Answer from the drawing. Dimensions are ordinates in mm from the lowest x, y and z of the part. Coordinates: 2 decimals unless noted, no trailing zeros. Order: outer loops, then holes, each group sorted by start corner. A loop starts at its lowest first (then second) coordinate and runs counter-clockwise, first axis right, second up.
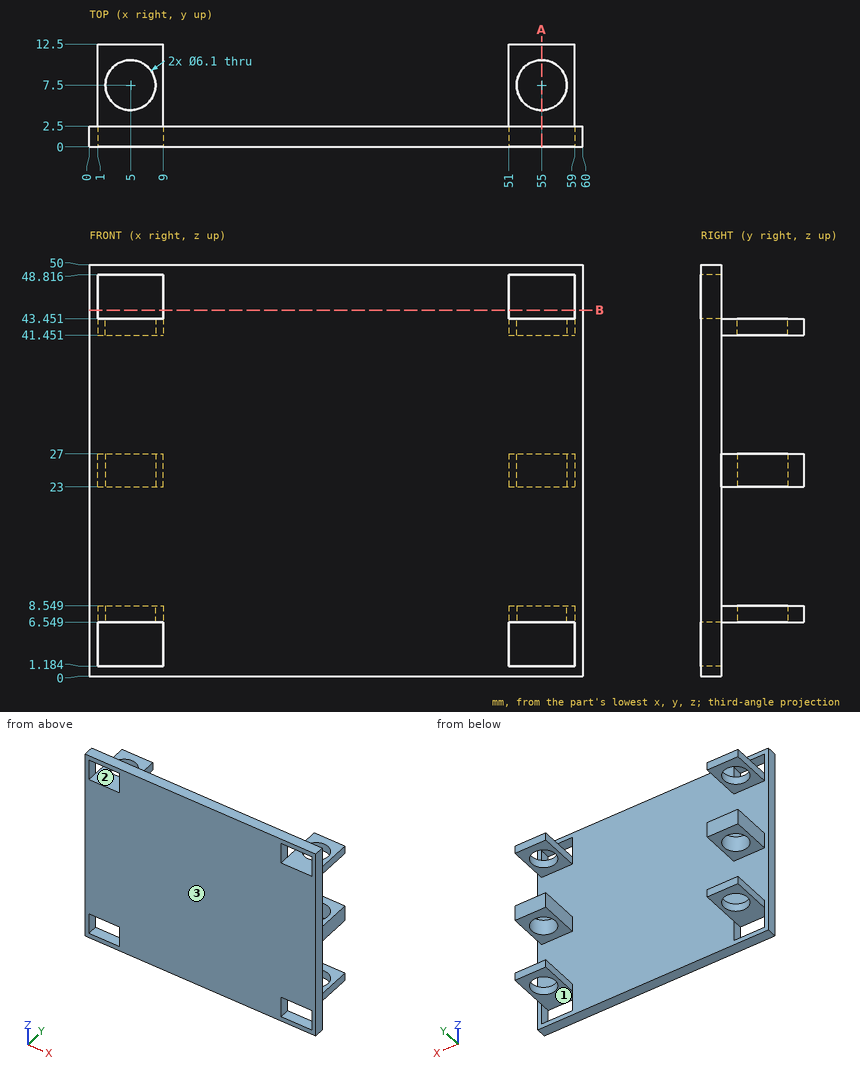
1) Determine the mould class of the marked faces 1, 2 and 3 for opening direction X: released by +X, released by -X, zero draft, split by the parting line, or undercut.
2) Each of these flat-tipped pins is pushed along its axis until it touches: P1, Ø1.2, axis at x = 3.5, y = 1, coming from the -Z side; P2, Ø2, axis at y = 8.5, z = 7, coming from the +X side; P3, Ø6.5, axis at x = 5, y = 7.5, coming from the -Z side; P4, Ø6.5, axis at x = 4, y = 7.5, coming from the +Z side. Where does it stop, or does it pass through?
3) Consider L1, parallel to Y at x = 55, z = 24.6; L2, parallel to Y at x = 16.5, z = 33; L3, parallel to Y at x = 54, z = 26. Determine where each line is inside the solid, lowest interval first.
4) Section B-B (z = 44.5) is taken. Give the vertices of the cut face in (x, y), then the cut area to 3 significant figures.
5) Section A-A (x = 55) is taken. Give the number of separate pieces and of enclosed holes in the cut face, then the cut area to 3 significant figures.
Filled sheet:
1. face 1: undercut
1. face 2: undercut
1. face 3: zero draft
2. P1: stops at z = 0
2. P2: stops at x = 59
2. P3: stops at z = 6.55
2. P4: stops at z = 43.45
3. L1: y = 0 to 4.45, 10.55 to 12.5
3. L2: y = 0 to 2.5
3. L3: y = 0 to 4.62, 10.38 to 12.5
4. outline: (0, 0) - (1, 0) - (1, 2.5) - (0, 2.5) - close; (9, 0) - (51, 0) - (51, 2.5) - (9, 2.5) - close; (59, 0) - (60, 0) - (60, 2.5) - (59, 2.5) - close
4. area: 110 mm2
5. separate pieces: 6
5. enclosed holes: 0
5. area: 129 mm2
